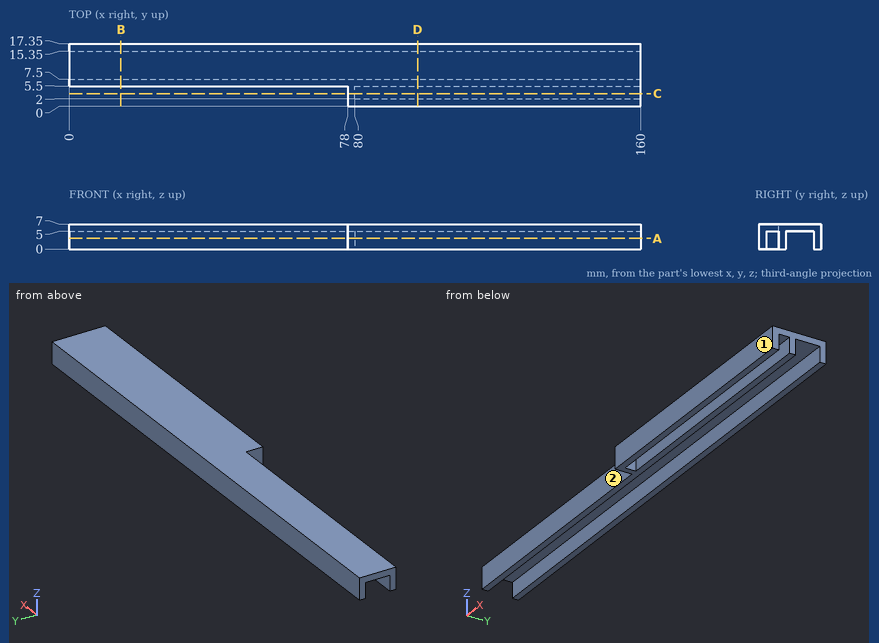
Geometry check sheet. Reference: drawing and pictorial views, mm from the part's lowest x, y, z. A direction names the side the tool comes from. Coordinates: 2 decimals unless noted, no trailing zeros. Order: outer loops, then holes, each group sorted by start corner. A loop starts at its lowest first (then second) coordinate and runs counter-clockwise, first axis right, second up.
Item 1: Tool access check on the marked faces 1 and 2. Record the directions out of +Z, -Z, +X, -X, +Y, -Y that give a thin tool (end or side, any length) a straight path to the whole face; none if there is none.
Item 2: Section check C-C (y = 3.5). Enter the section's corners in (x, z).
Item 3: Section check D-D (x = 97.5). Enter the section's corners in (y, z).
Item 4: Depth check by flat-ended pin: pin 1 (1 mm diameter, centred on y = 4, z = 2.5, fed in from +X); pin 2 (1 mm diameter, centred on x = 65, y = 12.5, fed in from -Z); pin 3 (3 mm diameter, centred on y = 3, z = 2, fed in from -X). Enter the tip coordinate at first touch or a pass-through.
Item 5: Section check B-B (x = 14.5). Enter the section's corners in (y, z), plus the area to 3 significant figures.
Item 6: Scan lines: line 1 along Y through (x, z) = (113, 3); line 2 along Y through (x, z) = (17, 0.5); line 3 along Y through (x, z) = (79.5, 2). Record each from-to range of solid material in increasing order.
Item 7: Section check A-A (z = 3). Enter the section's corners in (x, y).
Check sheet entries:
1. face 1: +Z, -Z, +X, -X, -Y
1. face 2: +Z, -Z, -X, -Y
2. outline: (78, 0) - (80, 0) - (80, 5) - (160, 5) - (160, 7) - (78, 7) - close
3. outline: (0, 0) - (2, 0) - (2, 5) - (5.5, 5) - (5.5, 0) - (7.5, 0) - (7.5, 5) - (15.35, 5) - (15.35, 0) - (17.35, 0) - (17.35, 7) - (0, 7) - close
4. pin 1: stops at x = 80
4. pin 2: stops at z = 5
4. pin 3: stops at x = 78
5. outline: (5.5, 0) - (7.5, 0) - (7.5, 5) - (15.35, 5) - (15.35, 0) - (17.35, 0) - (17.35, 7) - (5.5, 7) - close
5. area: 43.7 mm2
6. line 1: y = 0 to 2, 5.5 to 7.5, 15.35 to 17.35
6. line 2: y = 5.5 to 7.5, 15.35 to 17.35
6. line 3: y = 0 to 7.5, 15.35 to 17.35
7. outline: (0, 5.5) - (78, 5.5) - (78, 0) - (160, 0) - (160, 2) - (80, 2) - (80, 5.5) - (160, 5.5) - (160, 7.5) - (0, 7.5) - close; (0, 15.35) - (160, 15.35) - (160, 17.35) - (0, 17.35) - close
